Source: CAD feature listing. Evaluate the final solid. Frame: model axes, mm. Face numbers are marked on the shaded views. Coordinates: 2 decimals unless noted, no trailing zeros. Loops run counter-clockwise (first coordinate to the right, second up) from the corner with the lowest first, then second, coordinate; pieces in that order, holes last.
from build123d import *

# Parameters (mm, degrees)
F1_ANGLE = 128.431819
F2_R     = 12.7
F3_R     = 6.35
F4_DEPTH = 6.35
F5_R     = 5.842


with BuildPart() as f1:
    # F0 (on Front) → F1 (revolve, symmetric)
    with BuildSketch(Plane.XZ) as f1_sk:
        with BuildLine():
            Line((0, 3.803344), (0, 0))
            Line((0, 0), (44.595737, 0))
            ThreePointArc((44.595737, 0), (51.598835, 19.948952), (52.667361, 41.064404))
            ThreePointArc((52.667361, 41.064404), (46.444255, 46.055297), (38.652573, 47.765777))
            ThreePointArc((38.652573, 47.765777), (30.501858, 51.290272), (26.174091, 59.04441))
            ThreePointArc((26.174091, 59.04441), (24.968043, 81.890542), (32.653302, 103.439026))
            Line((32.653302, 103.439026), (28.97153, 103.439026))
            ThreePointArc((28.97153, 103.439026), (22.44019, 81.38567), (24.050664, 58.44193))
            ThreePointArc((24.050664, 58.44193), (29.180601, 49.206171), (38.813263, 44.867128))
            ThreePointArc((38.813263, 44.867128), (44.498632, 43.552613), (49.333733, 40.285632))
            ThreePointArc((49.333733, 40.285632), (48.862981, 21.585272), (43.055389, 3.803344))
            Line((43.055389, 3.803344), (0, 3.803344))
        make_face()
    revolve(axis=Axis((0, 0, 1.901672), (0, 0, -1)), revolution_arc=F1_ANGLE / 2)
    revolve(f1_sk.sketch, axis=Axis((0, 0, 1.901672), (0, 0, 1)), revolution_arc=F1_ANGLE / 2)

    # F2
    f2_edges = [f1.edges().sort_by_distance(p)[0] for p in [
        (44.61179, -27.993555, 41.064404),
    ]]
    fillet(f2_edges, radius=F2_R)

    # F3 (on face) → F4 (join)
    with BuildSketch(Plane(origin=(0, 0, 0), x_dir=(1, 0, 0), z_dir=(0, 0, -1))):
        with Locations((37.261488, 0)):
            Circle(F3_R)
    extrude(amount=F4_DEPTH)

    # F5
    f5_edges = [f1.edges().sort_by_distance(p)[0] for p in [
        (30.911488, 0, -6.35),
    ]]
    fillet(f5_edges, radius=F5_R)


solid = f1.part
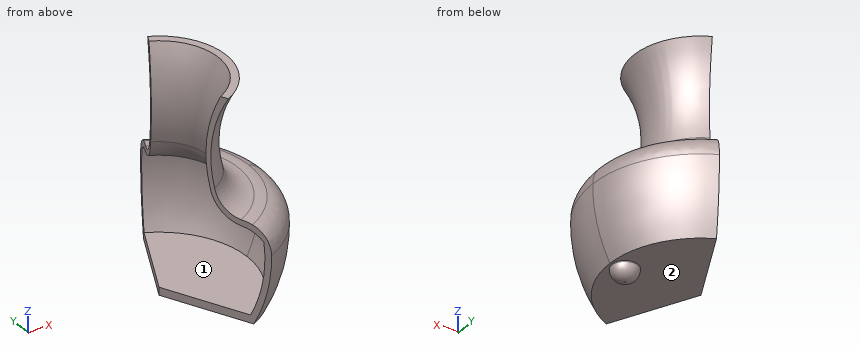
Q1. Section A-A, the plane z = 96. Return the cut outline in (x, y).
Q2. Section B-B, the plane z = 62.5. Return the cut outline in (x, y).
Q3. Draft query along Y for the marked faces 1 and 2. Return one class per face: +Y half, -Y half, draft (parallel to the pull), parting line (faces both ways), or undercut.
Q4. Contact query for flat-ended pins moving along their axis: pin 1 Ø12 at (y, z) = (13.5, 48) entering from -X; pin 2 Ø12 at (x, z) = (40, 8) entering from +Y; pin 3 Ø8 at (y, z) = (22.5, 79) entering from +X. Output: stop coordinate, or through.
Q5. Line query: line 1 along Z through (x, y) = (19.5, 23); line 2 along Z through (x, y) = (26.5, 11.5); line 3 along Z through (x, y) = (7.5, -7.5). Output: solid intervals per line, ascending.
Derived:
1. outline: (11.22, -23.22) - (12.57, -26.01) arc R28.89 ccw to (12.57, 26.01) - (11.22, 23.22) arc R25.79 cw to start
2. outline: (10.07, -20.85) - (11.05, -22.87) arc R25.4 ccw to (11.05, 22.87) - (10.07, 20.85) arc R23.16 cw to start
3. face 1: undercut
3. face 2: draft
4. pin 1: stops at x = 19.79
4. pin 2: stops at y = 34.87
4. pin 3: stops at x = 16.28
5. line 1: z = 0 to 3.8, 48.38 to 51.62, 98.81 to 103.44
5. line 2: z = 0 to 3.8, 49.48 to 53.02, 96 to 103.27
5. line 3: z = 0 to 3.8
